Source: CAD feature listing. Evaluate the final solid. Frame: model axes, mm. A direction names the side the tool comes from. Give positions to 0.01 mm unless a question says otherwise; leave off trailing zeros. Loops run counter-clockwise (first coordinate to the right, second up) from the corner with the lowest first, then second, coordinate; pieces in that order, holes last. Notation, with made-up numbers: (-18.5, 55) - (20.5, 55) arc R21 ccw to (20.5, 93) - close; hole circle Ø6 at (50.5, -25.75). An arc over 180 degrees is marked (long way). Put each result on its own line as item: value.
```python
from build123d import *

# Parameters (mm, degrees)
SKETCH1_R           = 9.3345
BOSS_EXTRUDE1_DEPTH = 0.8128
BOSS_EXTRUDE1_TAPER = 1
SKETCH2_R           = 7.5692
SKETCH3_R           = 7.7343
CIRPATTERN3_COUNT   = 24
FILLET1_R           = 0.508
SKETCH20_R          = 6.731
BOSS_EXTRUDE2_DEPTH = 13.1572
BOSS_EXTRUDE2_DRAFT = -2
SKETCH21_R          = 4.9657
CUT_EXTRUDE1_DEPTH  = 12.2174
SKETCH22_R          = 2.1971
CUT_EXTRUDE2_DEPTH  = 38.8968


with BuildPart() as part:
    # Sketch1 → Boss-Extrude1 (new body)
    with BuildSketch(Plane(origin=(0, 0, 0), x_dir=(1, 0, 0), z_dir=(0, 1, 0))):
        Circle(SKETCH1_R)
    extrude(amount=BOSS_EXTRUDE1_DEPTH, taper=BOSS_EXTRUDE1_TAPER)

    # Sketch2 → Loft1 section 0
    with BuildSketch(Plane(origin=(0, 13.6652, 0), x_dir=(1, 0, 0), z_dir=(0, 1, 0))):
        Circle(SKETCH2_R)
    # Sketch3 → Loft1 section 1
    with BuildSketch(Plane(origin=(0, 0.8128, 0), x_dir=(1, 0, 0), z_dir=(0, 1, 0))):
        Circle(SKETCH3_R)
    loft()

    # Sweep1: sweep along a path in Sketch4
    with BuildLine(Plane(origin=(0, 0, 0), x_dir=(0, 0, -1), z_dir=(1, 0, 0))) as sweep1_path:
        Line((-8.812312523, 0.8128), (-7.575725692, 13.1572))
    # Sketch14 → Sweep1 (sweep)
    with BuildSketch(Plane(origin=(0, 0.8128, 8.812312523), x_dir=(1, 0, 0), z_dir=(0, 0.995020042, -0.09967505))):
        Polygon((0, 0), (-0.711410859, 1.016), (0.711410859, 1.016), align=None)
    sweep1 = sweep(path=sweep1_path.line)

    # CirPattern3: Sweep1 ×24 about axis
    cirpattern3_axis = Axis((0, 0, 0), (0, 1, 0))
    for i in range(1, CIRPATTERN3_COUNT):
        add(sweep1.rotate(cirpattern3_axis, i * 360 / CIRPATTERN3_COUNT))

    # Sketch7 → Revolve1 (revolve)
    with BuildSketch(Plane(origin=(0, 0, 0), x_dir=(0, 0, -1), z_dir=(1, 0, 0))):
        with BuildLine():
            Line((6.6421, 18.415), (6.6167, 18.415))
            ThreePointArc((6.6167, 18.415), (5.0927, 16.0401), (6.6167, 13.6652))
            Line((6.6167, 13.6652), (0, 13.6652))
            Line((0, 13.6652), (0, 26.2128))
            Line((0, 26.2128), (6.6167, 26.2128))
            Line((6.6167, 26.2128), (6.6167, 24.765))
            ThreePointArc((6.6167, 24.765), (5.0927, 22.3901), (6.6167, 20.0152))
            Line((6.6167, 20.0152), (6.6421, 20.0152))
            Line((6.6421, 20.0152), (6.6421, 18.415))
        make_face()
    revolve(axis=Axis((0, 13.6652, 0), (0, 1, 0)))

    # Sketch19 → Cut-Revolve1 (revolve, cut)
    with BuildSketch(Plane(origin=(0, 0, 0), x_dir=(0, 0, -1), z_dir=(1, 0, 0))):
        Polygon((3.2004, 0), (3.412325434, 12.1412), (5.567182638, 12.1412), (6.6294, 0), (6.6294, -2.54), (3.2004, -2.54), align=None)
    revolve(axis=Axis((0, 0, 0), (0, 1, 0)), mode=Mode.SUBTRACT)

    # Fillet1
    fillet1_edges = [part.edges().sort_by_distance(p)[0] for p in [
        (-9.320312523, 0.8128, 0),
    ]]
    fillet(fillet1_edges, radius=FILLET1_R)


with BuildPart() as boss_extrude2_tool:
    # Sketch20 → Boss-Extrude2 (with draft: the straight prism first)
    with BuildSketch(Plane(origin=(0, 37.8968, 0), x_dir=(-1, 0, 0), z_dir=(0, -1, 0))):
        Circle(SKETCH20_R)
    extrude(amount=BOSS_EXTRUDE2_DEPTH)
    # Boss-Extrude2: the draft: its side faces are tilted about the plane it starts from
    boss_extrude2_sides = [boss_extrude2_tool.faces().sort_by_distance(p)[0] for p in [
        (6.731, 31.3182, 0),
    ]]
    draft(boss_extrude2_sides, Plane(origin=(0, 37.8968, 0), x_dir=(-1, 0, 0), z_dir=(0, -1, 0)), BOSS_EXTRUDE2_DRAFT)


with BuildPart() as part_1:
    add(part.part)

    # Boss-Extrude2: add boss_extrude2_tool
    add(boss_extrude2_tool.part)

    # Sketch21 → Cut-Extrude1 (cut)
    with BuildSketch(Plane(origin=(0, 37.8968, 0), x_dir=(1, 0, 0), z_dir=(0, 1, 0))):
        with Locations(Location((0, 0, 0), (0, 0, 270))):  # turned: the seam where the file's is
            Circle(SKETCH21_R)
    extrude(amount=-CUT_EXTRUDE1_DEPTH, mode=Mode.SUBTRACT)

    # Sketch22 → Cut-Extrude2 (cut, through all)
    with BuildSketch(Plane.XZ):
        with Locations(Location((0, 0, 0), (0, 0, 270))):  # turned: the seam where the file's is
            Circle(SKETCH22_R)
    extrude(amount=-CUT_EXTRUDE2_DEPTH, mode=Mode.SUBTRACT)


solid = part_1.part
```
1) Mould query, pull axis X, two halves, no side actions, for faces 1 (the flat face through (-0.28, 4.29, 8.06)), 2 (the flat face through (5.9, 4.29, -5.5)), 3 (the flat face through (-4.204, 5.661, -6.738)). Classes: pulls with the +X half, pulls with the -X half, needs draft (parallel to the pull), parting line crosses it, or undercut.
Check result:
face 1: undercut
face 2: pulls with the +X half
face 3: pulls with the -X half
2) Material intervals for line 1 along X through (y, z) = (7, 1.5); line 2 along Y through (x, z) = (1.25, 3.5); line 3 along X through (y, z) = (18.5, -1.25), sorted ascending. Write a range as [from, to].
Check result:
line 1: [-7.51, -5.83], [-2.96, -1.61], [1.61, 2.96], [5.83, 7.51]
line 2: [12.14, 25.68]
line 3: [-6.52, -1.81], [1.81, 6.52]
3) Pin query (flat end, axial travel): P1, Ø3, axis at y = 22, z = 7, coming from the -X side; P2, Ø8, axis at x = -1.5, y = 30.5, coming from the -Z side; P3, Ø4, axis at x = -1.5, y = 24, coming from the -Z side; P4, Ø4, axis at x = 5.5, y = 17, coming from the -Z side. Return the tip coordinate at first contact, or that it passes through.
Check result:
P1: through
P2: z = -7.12
P3: z = -7.19
P4: z = -5.24
4) Access query for faces 4 (the flat face through (-1.03, 25.679, 2.14)), 5 (the flat face through (-5.8, 5.7, -5.4)), 6 (the flat face through (4.204, 5.661, 6.738)). Directions: +Z, -Z, +X, -X, +Y, -Y. A direction counts if a zero-diameter tool reaches every point of the face in a straight line with its end or side. Return the directions, or none.
Check result:
face 4: +Y
face 5: -X, +Y
face 6: +Z, +X, +Y
5) Section query B-B, the plane y = 19. Output: boundary loops of the cut face in (x, z), plus the area to 3 significant figures.
Check result:
outline: circle Ø13.28 at (0, 0); hole circle Ø4.39 at (0, 0)
area: 123 mm²
6) Section query A-A, the plane y = 29. Output: boundary loops of the cut face in (x, z), plus the area to 3 significant figures.
Check result:
outline: circle Ø14.08 at (0, 0); hole circle Ø9.93 at (0, 0)
area: 78.3 mm²
